Could you check a few things on this model? Use its own coordinates, in mm. A direction names the side the tool comes from. Give positions to 0.01 mm unless a question says otherwise; leave off trailing zeros. Loops run counter-clockwise (first coordinate to the right, second up) from the corner with the lowest first, then second, coordinate; pieces in that order, holes last. Notation, with made-up numbers: (89.25, 63) - (126.25, 63) arc R21 cw to (126.25, 68) - close; hole circle Ø5 at (-30, 51). An arc over 180 degrees is marked (long way). Answer in a Markdown table with one row per item. Add a question column.
```python
from build123d import *

# Parameters (mm, degrees)
SKETCH002_W     = 79.5
SKETCH002_H     = 104
SKETCH002_R     = 1.5
PAD002_DEPTH    = 12.5
SKETCH_W        = 8.021301
SKETCH_H        = 8.234894
SKETCH_R        = 1.5
PAD_DEPTH       = 2.5
POCKET_DEPTH    = 2
SKETCH033_W     = 7.946812
SKETCH033_H     = 7.946812
SKETCH033_R     = 1.5
PAD003_DEPTH    = 3
SKETCH034_W     = 6.801386
SKETCH034_H     = 103.670945
SKETCH034_R     = 1.5
PAD004_DEPTH    = 3
POCKET001_DEPTH = 2
POCKET002_DEPTH = 2
POCKET003_DEPTH = 2
POCKET027_DEPTH = 0.5


with BuildPart() as part:
    # Sketch002 → Pad002 (new body)
    with BuildSketch(Plane.XY):
        with Locations((-2.25, 6.5)):
            Rectangle(SKETCH002_W, SKETCH002_H)
        with Locations((-38.5, 55)):
            Circle(SKETCH002_R, mode=Mode.SUBTRACT)
        with Locations((34, 55)):
            Circle(SKETCH002_R, mode=Mode.SUBTRACT)
        with Locations((-38.5, -42)):
            Circle(SKETCH002_R, mode=Mode.SUBTRACT)
        with Locations((34, -42)):
            Circle(SKETCH002_R, mode=Mode.SUBTRACT)
        with BuildLine():
            Line((34, -45), (-38.5, -45))
            ThreePointArc((-38.5, -45), (-36.37868, -39.87868), (-41.5, -42))
            Line((-41.5, -42), (-41.5, 55))
            ThreePointArc((-41.5, 55), (-36.37868, 52.87868), (-38.5, 58))
            Line((-38.5, 58), (34, 58))
            ThreePointArc((34, 58), (31.87868, 52.87868), (37, 55))
            Line((37, 55), (37, -42))
            ThreePointArc((37, -42), (31.87868, -39.87868), (34, -45))
        make_face(mode=Mode.SUBTRACT)
    extrude(amount=-PAD002_DEPTH)

    # Sketch → Pad (join)
    with BuildSketch(Plane.XY):
        with Locations((-37.87762, 47.077984)):
            Rectangle(SKETCH_W, SKETCH_H)
        with Locations((-37.997646, 47.010536)):
            Circle(SKETCH_R, mode=Mode.SUBTRACT)
    extrude(amount=-PAD_DEPTH)

    # Sketch032 (on Face23 of Pad) → Pocket (cut)
    with BuildSketch(Plane.XY):
        Polygon((-34.726036, 46.982567), (-36.351036, 49.79715), (-39.601036, 49.79715), (-41.226036, 46.982567), (-39.601036, 44.167984), (-36.351036, 44.167984), align=None)
    extrude(amount=-POCKET_DEPTH, mode=Mode.SUBTRACT)

    # Sketch033 → Pad003 (join)
    with BuildSketch(Plane.XY):
        with Locations((-37.923063, -11.232048)):
            Rectangle(SKETCH033_W, SKETCH033_H)
        with Locations((-37.99107, -11.008605)):
            Circle(SKETCH033_R, mode=Mode.SUBTRACT)
    extrude(amount=-PAD003_DEPTH)

    # Sketch034 → Pad004 (join)
    with BuildSketch(Plane.XY):
        with Locations((10.981288, 6.512218)):
            Rectangle(SKETCH034_W, SKETCH034_H)
        with Locations((11.033937, 47.026531)):
            Circle(SKETCH034_R, mode=Mode.SUBTRACT)
        with Locations((11.033937, -10.967275)):
            Circle(SKETCH034_R, mode=Mode.SUBTRACT)
    extrude(amount=-PAD004_DEPTH)

    # Sketch035 (on Face34 of Pad004) → Pocket001 (cut)
    with BuildSketch(Plane.XY):
        Polygon((-36.326836, -8.14599), (-39.576836, -8.14599), (-41.201836, -10.960573), (-39.576836, -13.775156), (-36.326836, -13.775156), (-34.701836, -10.960573), align=None)
    extrude(amount=-POCKET001_DEPTH, mode=Mode.SUBTRACT)

    # Sketch036 (on Face26 of Pocket001) → Pocket002 (cut)
    with BuildSketch(Plane.XY):
        Polygon((12.678073, 49.85376), (9.428073, 49.85376), (7.803073, 47.039177), (9.428073, 44.224594), (12.678073, 44.224594), (14.303073, 47.039177), align=None)
    extrude(amount=-POCKET002_DEPTH, mode=Mode.SUBTRACT)

    # Sketch037 (on Face26 of Pocket002) → Pocket003 (cut)
    with BuildSketch(Plane.XY):
        Polygon((12.636199, -8.121596), (9.386199, -8.121596), (7.761199, -10.936179), (9.386199, -13.750762), (12.636199, -13.750762), (14.261199, -10.936179), align=None)
    extrude(amount=-POCKET003_DEPTH, mode=Mode.SUBTRACT)

    # Sketch058 → Pocket027 (cut)
    with BuildSketch(Plane.YZ.offset(37)):
        with BuildLine():
            ThreePointArc((-14.544005, 0.366508), (-16.544005, -1.633492), (-14.544005, -3.633492))
            Line((-14.544005, -3.633492), (-6.544005, -3.633492))
            ThreePointArc((-6.544005, -3.633492), (-4.544005, -1.633492), (-6.544005, 0.366508))
            Line((-6.544005, 0.366508), (-14.544005, 0.366508))
        make_face()
        with BuildLine():
            ThreePointArc((19.455995, 0.366508), (17.455995, -1.633492), (19.455995, -3.633492))
            Line((19.455995, -3.633492), (27.455995, -3.633492))
            ThreePointArc((27.455995, -3.633492), (29.455995, -1.633492), (27.455995, 0.366508))
            Line((27.455995, 0.366508), (19.455995, 0.366508))
        make_face()
    extrude(amount=POCKET027_DEPTH, mode=Mode.SUBTRACT)


solid = part.part
```
(1) I want a section at D-D on y = 25. Please give me the cut outline in (x, z), then the cut area to 3 significant figures.
(2) I want a section at B-B on x = -10.5. Please give me the cut outline in (y, z), then the cut area to 3 significant figures.
(3) I want a section at A-A on y = 0. Please give me the cut outline in (x, z).
(4) Please list where these lines run through material, in increasing order: line 1 (X direction, y = -35, z = -1.75); line 2 (Y direction, x = -19, z = -10.75); line 3 (X direction, y = -1, z = -11.25).
(5) On a 3-axis mill with a long thin cutter (end or side, diameter ignored), from which of +Z, -Z, +X, -X, +Y, -Y can I reach the whole of each face in a straight line? I mean faces 3 (the cylindrical face through (37.25, 29.35, -2.27)), 4 (the flat face through (33, 53, -12.5)), 5 (the flat face through (12.5, 48.3, -2)), 6 (the flat face through (-38, -15.205, -1)). Say none if no direction works.
(6) For pin 1 Ø1.8 at (x, y) = (11.03, 47.03) entering from -Z; pin 2 Ø2.5 at (y, z) = (-8.5, -1.5) entering from +X; pin 3 Ø1.7 at (x, y) = (-38.5, 47.5) entering from +Z; pin 4 Ø5 at (x, y) = (9, 2.5) entering from -Z, each with a flat end and sliding along its axis, tell me the tip position at first contact or that it passes through.
(7) I want a section at C-C on z = -10. Please give me the cut outline in (x, y), then the cut area to 3 significant figures.
(8) We'd pull the mould along Y, two halves only. Please class faces 1 (the flat face through (9, 7, 0)), 2 (the flat face through (11, 44.225, -1)): pulls with the +Y half, pulls with the -Y half, needs draft (parallel to the pull), parting line crosses it, or undercut.
Reported:
| question | item | result |
|---|---|---|
| 1 | outline | (-42, -12.5) - (-41.5, -12.5) - (-41.5, 0) - (-42, 0) - close; (7.58, -3) - (14.38, -3) - (14.38, 0) - (7.58, 0) - close; (37, -12.5) - (37.5, -12.5) - (37.5, -3.63) - (37, -3.63) - close |
| 1 | area | 31.1 mm² |
| 2 | outline | (-45.5, -12.5) - (-45, -12.5) - (-45, 0) - (-45.5, 0) - close; (58, -12.5) - (58.5, -12.5) - (58.5, 0) - (58, 0) - close |
| 2 | area | 12.5 mm² |
| 3 | outline | (-42, -12.5) - (-41.5, -12.5) - (-41.5, 0) - (-42, 0) - close; (7.58, -3) - (14.38, -3) - (14.38, 0) - (7.58, 0) - close; (37, -12.5) - (37.5, -12.5) - (37.5, 0) - (37, 0) - close |
| 4 | line 1 | -42 to -41.5, 7.58 to 14.38, 37 to 37.5 |
| 4 | line 2 | -45.5 to -45, 58 to 58.5 |
| 4 | line 3 | -42 to -41.5, 37 to 37.5 |
| 5 | face 3 | +X |
| 5 | face 4 | -Z, +X, -X, +Y, -Y |
| 5 | face 5 | +Z |
| 5 | face 6 | +Z, -Z |
| 6 | pin 1 | through |
| 6 | pin 2 | x = 14.38 |
| 6 | pin 3 | z = -2 |
| 6 | pin 4 | z = -3 |
| 7 | outline | (-42, -45.5) - (37.5, -45.5) - (37.5, 58.5) - (-42, 58.5) - close; hole (-41.5, -42) arc R3 cw (long way) to (-38.5, -45) - (34, -45) arc R3 cw (long way) to (37, -42) - (37, 55) arc R3 cw (long way) to (34, 58) - (-38.5, 58) arc R3 cw (long way) to (-41.5, 55) - close; hole circle Ø3 at (-38.5, -42); hole circle Ø3 at (-38.5, 55); hole circle Ø3 at (34, -42); hole circle Ø3 at (34, 55) |
| 7 | area | 275 mm² |
| 8 | face 1 | needs draft |
| 8 | face 2 | undercut |
